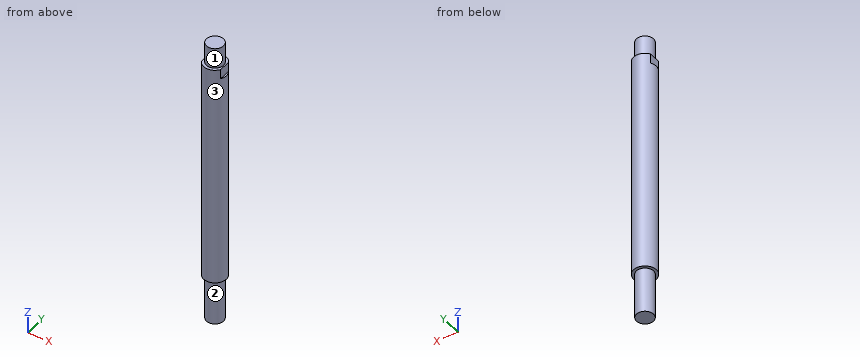
from build123d import *

# Parameters (mm, degrees)
SKETCH1_R           = 20
BOSS_EXTRUDE1_DEPTH = 255
SKETCH2_R           = 20
SKETCH2_R_2         = 15
CUT_EXTRUDE1_DEPTH  = 36
SKETCH3_W           = 9.924415088
SKETCH3_H           = 50.469281605
SKETCH3_W_2         = 14.039416466
SKETCH3_H_2         = 45.628103513
CUT_EXTRUDE2_DEPTH  = 17
CUT_EXTRUDE4_START  = -80
SKETCH4_R           = 20
SKETCH4_R_2         = 15
CUT_EXTRUDE4_DEPTH  = 80


with BuildPart() as part:
    # Sketch1 → Boss-Extrude1 (new, symmetric)
    with BuildSketch(Plane.XY):
        Circle(SKETCH1_R)
    extrude(amount=BOSS_EXTRUDE1_DEPTH, both=True)

    # Sketch2 → Cut-Extrude1 (cut)
    with BuildSketch(Plane.XY.offset(255)):
        Circle(SKETCH2_R)
        Circle(SKETCH2_R_2, mode=Mode.SUBTRACT)
    extrude(amount=-CUT_EXTRUDE1_DEPTH, mode=Mode.SUBTRACT)

    # Sketch3 → Cut-Extrude2 (cut)
    with BuildSketch(Plane.XY.offset(219)):
        with Locations((-21.962207544, 3.05599367)):
            Rectangle(SKETCH3_W, SKETCH3_H)
        with Locations((24.019708233, 0.635404624)):
            Rectangle(SKETCH3_W_2, SKETCH3_H_2)
    extrude(amount=-CUT_EXTRUDE2_DEPTH, mode=Mode.SUBTRACT)

    # Sketch4 → Cut-Extrude4 (cut)
    with BuildSketch(Plane(origin=(0, 0, -255), x_dir=(-1, 0, 0), z_dir=(0, 0, -1)).offset(CUT_EXTRUDE4_START)):
        Circle(SKETCH4_R)
        with Locations(Location((0, 0, 0), (0, 0, 180))):
            Circle(SKETCH4_R_2, mode=Mode.SUBTRACT)
    extrude(amount=CUT_EXTRUDE4_DEPTH, mode=Mode.SUBTRACT)


solid = part.part
Work out the finished part from the listing and answer in its coordinate system (mm). Face numbers are marked on the shaded views. A direction names the side the tool comes from. Round coordinates to 2 decimals unless told otherwise and drop trailing zeros. Order: outer loops, then holes, each group sorted by start corner. A loop starts at its lowest first (then second) coordinate and runs counter-clockwise, first axis right, second up. Notation, with made-up numbers: M 54,56 L 91,56 A26 ccw 91,74 Z; hole C 7.25,39.25 d11. An arc over 180 degrees is marked long. Put each result on its own line as item: value. Start each with the question number.
Q1. A tool of negligible diameter and unlimited length cuts with its end or side. For the marked faces 1, 2 and 3, from which of +Z, -Z, +X, -X, +Y, -Y can it reach the whole face along a straight path? Write none if from no direction.
Q2. Section C-C, the plane z = -79 is taken. Write down the section's boundary in (x, y), and give its area (3 significant figures).
Q3. Straight lines are drawn through the part: L1, parallel to Y at x = -1.5, z = 101; L2, parallel to Y at x = 1, z = 162.5; L3, parallel to Z at x = 12.5, y = 11. For each, find the intervals that lie inside material, in ascending order. Write a range as [from, to].
Q4. Section A-A, the plane x = 0 is taken. Write down the section's boundary in (y, z).
Q5. Section B-B, the plane y = 0 is taken. Write down the section's boundary in (x, z).
Q6. Flat-ended cylindrical pins translate along their axes: pin 1 (3.5 mm diameter, centred on x = -18, y = -1.5, fed in from +Z); pin 2 (2 mm diameter, centred on y = 14.5, z = 138.5, fed in from -X); pin 3 (5 mm diameter, centred on y = 3, z = 212, fed in from -X). Find the tip coordinate at first contact, or state that the pin passes through.
Findings below:
1. face 1: +Z
1. face 2: -Z
1. face 3: +Z, -Z
2. outline: C 0,0 d40
2. area: 1,260 mm^2
3. L1: y = [-19.94, 19.94]
3. L2: y = [-19.97, 19.97]
3. L3: z = [-175, 219]
4. outline: M -20,-175 L -15,-175 L -15,-255 L 15,-255 L 15,-175 L 20,-175 L 20,219 L 15,219 L 15,255 L -15,255 L -15,219 L -20,219 Z
5. outline: M -20,-175 L -15,-175 L -15,-255 L 15,-255 L 15,-175 L 20,-175 L 20,202 L 17,202 L 17,219 L 15,219 L 15,255 L -15,255 L -15,219 L -17,219 L -17,202 L -20,202 Z
6. pin 1: stops at z = 219
6. pin 2: stops at x = -14.76
6. pin 3: stops at x = -17
